from build123d import *

# Parameters (mm, degrees)
SKETCH1_W                 = 58
SKETCH1_H                 = 24
BOSS_EXTRUDE1_DEPTH       = 28.3
SKETCH2_W                 = 88
SKETCH2_H                 = 68
BOSS_EXTRUDE2_DEPTH       = 2
SKETCH12_W                = 41.2
SKETCH12_H                = 20.2
CUT_EXTRUDE1_DEPTH        = 27.95
BOSS_EXTRUDE6_DEPTH       = 2
LPATTERN2_COUNT           = 3
LPATTERN2_PITCH           = 28
BOSS_EXTRUDE7_DEPTH       = 2
LPATTERN3_COUNT           = 2
LPATTERN3_PITCH           = 22
SKETCH17_R                = 1
CUT_EXTRUDE2_DEPTH        = 10
F_8_32_TAPPED_HOLE1_D     = 3.4544
F_8_32_TAPPED_HOLE1_DEPTH = 12
F_8_32_TAPPED_HOLE1_TIP   = 1.037806461
FILLET1_R                 = 15
FILLET2_R                 = 15
FILLET3_R                 = 15
FILLET5_R                 = 15
SKETCH20_W                = 16
SKETCH20_H                = 23.3
CUT_EXTRUDE3_DEPTH        = 10
SKETCH21_W                = 16
SKETCH21_H                = 23.3
CUT_EXTRUDE4_DEPTH        = 10
FILLET6_R                 = 4
FILLET7_R                 = 4
FILLET8_R                 = 4
FILLET9_R                 = 4


with BuildPart() as part:
    # Sketch1 → Boss-Extrude1 (new body)
    with BuildSketch(Plane(origin=(0, 0, 0), x_dir=(1, 0, 0), z_dir=(0, 1, 0))):
        Rectangle(SKETCH1_W, SKETCH1_H)
    extrude(amount=BOSS_EXTRUDE1_DEPTH)

    # Sketch2 → Boss-Extrude2 (add)
    with BuildSketch(Plane.XZ):
        Rectangle(SKETCH2_W, SKETCH2_H)
    extrude(amount=BOSS_EXTRUDE2_DEPTH)

    # Sketch12 → Cut-Extrude1 (cut)
    with BuildSketch(Plane(origin=(0, 28.3, 0), x_dir=(1, 0, 0), z_dir=(0, 1, 0))):
        Rectangle(SKETCH12_W, SKETCH12_H)
    extrude(amount=-CUT_EXTRUDE1_DEPTH, mode=Mode.SUBTRACT)

    # Sketch14 → Boss-Extrude6 (add)
    with BuildSketch(Plane.ZY.offset(29)):
        Polygon((-12, 28.3), (-12, 0), (-34, 0), align=None)
        Polygon((12, 28.3), (12, 0), (34, 0), align=None)
    boss_extrude6 = extrude(amount=-BOSS_EXTRUDE6_DEPTH)

    # LPattern2: Boss-Extrude6 ×3
    with Locations(*[(i * LPATTERN2_PITCH, 0, 0) for i in range(1, LPATTERN2_COUNT)]):
        add(boss_extrude6)

    # Sketch16 → Boss-Extrude7 (add)
    with BuildSketch(Plane(origin=(0, 0, -12), x_dir=(-1, 0, 0), z_dir=(0, 0, -1))):
        Polygon((-29, 28.3), (-44, 0), (-29, 0), align=None)
        Polygon((29, 28.3), (29, 0), (44, 0), align=None)
    boss_extrude7 = extrude(amount=-BOSS_EXTRUDE7_DEPTH)

    # LPattern3: Boss-Extrude7 ×2
    with Locations(*[(0, 0, i * LPATTERN3_PITCH) for i in range(1, LPATTERN3_COUNT)]):
        add(boss_extrude7)

    # Sketch17 → Cut-Extrude2 (cut)
    with BuildSketch(Plane(origin=(0, 28.3, 0), x_dir=(1, 0, 0), z_dir=(0, 1, 0))):
        with Locations(Location((-24.4, 5, 0), (0, 0, 270))):
            Circle(SKETCH17_R)
        with Locations(Location((-24.4, -5, 0), (0, 0, 270))):
            Circle(SKETCH17_R)
        with Locations(Location((24.4, -5, 0), (0, 0, 270))):
            Circle(SKETCH17_R)
        with Locations(Location((24.4, 5, 0), (0, 0, 270))):
            Circle(SKETCH17_R)
    extrude(amount=-CUT_EXTRUDE2_DEPTH, mode=Mode.SUBTRACT)

    # #8-32 Tapped Hole1
    with Locations(Plane(origin=(-24.4, 28.3, -5), x_dir=(0, 0, 1), z_dir=(0, 1, 0))):
        with Locations((0, 0), (10, 0), (0, 48.8), (10, 48.8)):
            Hole(F_8_32_TAPPED_HOLE1_D / 2, depth=F_8_32_TAPPED_HOLE1_DEPTH)
            with Locations((0, 0, -(F_8_32_TAPPED_HOLE1_DEPTH + F_8_32_TAPPED_HOLE1_TIP / 2))):  # 118° drill point
                Cone(0, F_8_32_TAPPED_HOLE1_D / 2, F_8_32_TAPPED_HOLE1_TIP, mode=Mode.SUBTRACT)

    # Fillet1
    fillet1_edges = [part.edges().sort_by_distance(p)[0] for p in [
        (-44, -1, 34),
    ]]
    fillet(fillet1_edges, radius=FILLET1_R)

    # Fillet2
    fillet2_edges = [part.edges().sort_by_distance(p)[0] for p in [
        (44, -1, 34),
    ]]
    fillet(fillet2_edges, radius=FILLET2_R)

    # Fillet3
    fillet3_edges = [part.edges().sort_by_distance(p)[0] for p in [
        (44, -1, -34),
    ]]
    fillet(fillet3_edges, radius=FILLET3_R)

    # Fillet5
    fillet5_edges = [part.edges().sort_by_distance(p)[0] for p in [
        (-44, -1, -34),
    ]]
    fillet(fillet5_edges, radius=FILLET5_R)

    # Sketch20 → Cut-Extrude3 (cut)
    with BuildSketch(Plane.ZY.offset(29)):
        with Locations((0, 14.65)):
            Rectangle(SKETCH20_W, SKETCH20_H)
    extrude(amount=-CUT_EXTRUDE3_DEPTH, mode=Mode.SUBTRACT)

    # Sketch21 → Cut-Extrude4 (cut)
    with BuildSketch(Plane(origin=(29, 0, 0), x_dir=(0, 0, -1), z_dir=(1, 0, 0))):
        with Locations((0, 14.65)):
            Rectangle(SKETCH21_W, SKETCH21_H)
    extrude(amount=-CUT_EXTRUDE4_DEPTH, mode=Mode.SUBTRACT)

    # Fillet6
    fillet6_edges = [part.edges().sort_by_distance(p)[0] for p in [
        (24.8, 3, 8),
    ]]
    fillet(fillet6_edges, radius=FILLET6_R)

    # Fillet7
    fillet7_edges = [part.edges().sort_by_distance(p)[0] for p in [
        (24.8, 3, -8),
    ]]
    fillet(fillet7_edges, radius=FILLET7_R)

    # Fillet8
    fillet8_edges = [part.edges().sort_by_distance(p)[0] for p in [
        (-24.8, 3, -8),
    ]]
    fillet(fillet8_edges, radius=FILLET8_R)

    # Fillet9
    fillet9_edges = [part.edges().sort_by_distance(p)[0] for p in [
        (-24.8, 3, 8),
    ]]
    fillet(fillet9_edges, radius=FILLET9_R)


solid = part.part
Work out the finished part from the listing and answer in its coordinate system (mm). A direction names the side the tool comes from. Coordinates: 2 decimals unless noted, no trailing zeros. Write each loop counter-clockwise with the first axis right and the second up, starting at its lowest first coordinate (ties: lowest second). Pieces come first, ordered by that corner, then holes. Notation, with made-up numbers: (-23.75, 6.25) - (1.25, 6.25) arc R9 ccw to (1.25, 21.25) - close; hole circle Ø9 at (37.5, -37.75). An arc over 180 degrees is marked (long way). One line per question, with ' | ' between items.
1) Consider probe 1 along X at (y, z) = (8.5, 26.5); probe 2 along X at (y, z) = (27, 5); probe 3 along Z at (x, y) = (8, 24). Determine where each line is inside the solid, lowest interval first. Write a range as [from, to].
Checks:
probe 1: [-29, -27], [-1, 1], [27, 29] | probe 2: [-29, -26.13], [-22.67, -20.6], [20.6, 22.67], [26.13, 29] | probe 3: [-12, -10.1], [10.1, 12]
2) The mould has two halves that part along X. Classify faces 1 (the face through (-39.49, -1.01, 29.72)), 2 (the face through (36.395, 14.348, 10.986)), 3 (the face through (14, 0, 23)), 4 (the face through (-24.741, 4.141, 6.797)): +X half, -X half, draft (parallel to the pull), parting line (faces both ways), or undercut.
Checks:
face 1: -X half | face 2: +X half | face 3: undercut | face 4: draft
3) Find section B-B, the plane x = 15. Determine the outline of the cut face in (y, z).
Checks:
outline: (-2, -34) - (0, -34) - (0, -12) - (28.3, -12) - (28.3, -10.1) - (0.35, -10.1) - (0.35, 10.1) - (28.3, 10.1) - (28.3, 12) - (0, 12) - (0, 34) - (-2, 34) - close
4) For faces 5 (the face through (25, 26.3, 0)), 6 (the face through (36, 0, -23)), 7 (the face through (-37, 0, -23)), 8 (the face through (22.714, 27.286, -4.626)), 9 (the face through (-33, 8, 10)), determine the directions among +Z, -Z, +X, -X, +Y, -Y from which every point of the face is accessible in a straight line to the end or side of a thin tool.
Checks:
face 5: +X, -X | face 6: -Z, +X, +Y | face 7: -Z, -X, +Y | face 8: +Y | face 9: -X, +Y
5) Find section D-D, the plane z = -14. Determine the outline of the cut face in (x, y), and give its area (3 significant figures).
Checks:
outline: (-44, -2) - (44, -2) - (44, 0) - (29, 0) - (29, 25.73) - (27, 25.73) - (27, 0) - (1, 0) - (1, 25.73) - (-1, 25.73) - (-1, 0) - (-27, 0) - (-27, 25.73) - (-29, 25.73) - (-29, 0) - (-44, 0) - close | area: 330 mm2
6) Find section A-A, the plane x = 24.4. Determine the outline of the cut face in (y, z), and give its area (3 significant figures).
Checks:
outline: (-2, -34) - (0, -34) - (0, -12) - (28.3, -12) - (28.3, -6.73) - (26.3, -6.73) - (26.3, -8) - (7, -8) arc R4 cw to (3, -4) - (3, 4) arc R4 cw to (7, 8) - (26.3, 8) - (26.3, 6.73) - (28.3, 6.73) - (28.3, 12) - (0, 12) - (0, 34) - (-2, 34) - close; (26.3, -3.27) - (28.3, -3.27) - (28.3, 3.27) - (26.3, 3.27) - close | area: 435 mm2
7) Flat-ended cylindrical pins translate along their axes: P1, Ø3, axis at x = -6.5, z = -6.5, coming from the +Y side; P2, Ø6.5, axis at x = 26.5, y = 13, coming from the +Z side; P3, Ø12, axis at y = 18, z = 27, coming from the -X side; P4, Ø10, axis at y = 10, z = -2, coming from the +X side. Find the tip coordinate at first contact, or state that the pin passes through.
Checks:
P1: y = 0.35 | P2: z = 26.39 | P3: x = -29 | P4: through
8) Find section C-C, the plane z = -5. Determine the outline of the cut face in (x, y).
Checks:
outline: (-44, -2) - (44, -2) - (44, 0) - (29, 0) - (29, 3.13) - (20.6, 3.13) - (20.6, 0.35) - (-20.6, 0.35) - (-20.6, 3.13) - (-29, 3.13) - (-29, 0) - (-44, 0) - close; (-29, 26.3) - (-26.13, 26.3) - (-26.13, 28.3) - (-29, 28.3) - close; (-22.67, 26.3) - (-20.6, 26.3) - (-20.6, 28.3) - (-22.67, 28.3) - close; (20.6, 26.3) - (22.67, 26.3) - (22.67, 28.3) - (20.6, 28.3) - close; (26.13, 26.3) - (29, 26.3) - (29, 28.3) - (26.13, 28.3) - close
